Verification items for the finished model (mm, model axes). A direction names the side the tool comes from. Give positions to 0.01 mm unless a question says otherwise; leave off trailing zeros. Write each loop counter-clockwise with the first axis right and the second up, starting at its lowest first coordinate (ties: lowest second). Pieces come first, ordered by that corner, then holes. Notation, with made-up numbers: (79, 32) -> (138, 32) arc R31 ccw to (138, 65) -> close; hole circle Ø5 at (-39, -17.5). An arc over 180 degrees is marked (long way). Answer as CSV lines item,"result". Start each with the question number.
1) Material ranges on L1, parallel to Y at x = 34, z = -106.5; L2, parallel to Z at x = -22.5, y = 29, recorded low to high.
2) Sectioned sample at A-A on x = -19.5. Record the cut outline in (y, z), and give its area (3 significant figures).
3) Sectioned sample at B-B on y = 19. Record the cut outline in (x, z) (1 decimal).
4) Tool access check on faces 4 (the flat face through (0, 98, 48)), 5 (the flat face through (-31.8, -3.1, -146)), 6 (the flat face through (3.175, 98, 48)). Record the directions out of +Z, -Z, +X, -X, +Y, -Y that give a thin tool (end or side, any length) a straight path to the whole face; none if there is none.
5) Sectioned sample at C-C on z = 17. Record the cut outline in (x, y) (3 decimals), and give its area (3 significant figures).
6) Sectioned sample at D-D on z = -62.5. Record the cut outline in (x, y) (3 decimals), and give its area (3 significant figures).
7) Mould release check, pull along Y, two halves, no side actions. Record for faces 1 (the flat face through (31.7, -3.1, -146.1)), 2 (the flat face through (1.565, 80.451, 67.685)), 3 (the flat face through (-1, -6.35, 2)): released by +Y, released by -Y, zero draft, split by the parting line, or undercut.
8) Gauge pin test, flat ends, axial feed: pin 1 Ø2 at (x, y) = (-30.5, 119.5) entering from -Z; pin 2 Ø6 at (x, z) = (23, -87.5) entering from +Y; pin 3 Ø4 at (x, y) = (27.5, 221) entering from +Z. Record the tip position at first contact, or that the pin passes through.
```python
from build123d import *

# Parameters (mm, degrees)
F1_DEPTH = 6.35
F3_W     = 304.8
F3_H     = 6.35
F4_DEPTH = 76.2
F6_DEPTH = 3.175
F7_DEPTH = 3.175


with BuildPart() as f1:
    # F0 (on Front) → F1 (new body)
    with BuildSketch(Plane.XZ):
        Polygon((-25.4, -152.4), (25.4, -152.4), (38.1, -139.7), (38.1, 152.4), (-38.1, 152.4), (-38.1, -139.7), align=None)
    extrude(amount=F1_DEPTH)

    # F3 (on offset) → F4 (join)
    with BuildSketch(Plane.YZ.offset(38.1)):
        with Locations((152.4, 149.089498)):
            Rectangle(F3_W, F3_H)
    extrude(amount=-F4_DEPTH)

    # F5 (on Right) → F6 (join)
    with BuildSketch(Plane.YZ):
        Polygon((0, -66.648165), (212.562662, 145.914498), (158.681126, 145.914498), (0, -12.766628), align=None)
    extrude(amount=F6_DEPTH)

    # F5 (on Right) → F7 (join)
    with BuildSketch(Plane.YZ):
        Polygon((0, -66.648165), (212.562662, 145.914498), (158.681126, 145.914498), (0, -12.766628), align=None)
    extrude(amount=F7_DEPTH)


solid = f1.part
```
Ans:
1,L1,"y = -6.35 to 0"
1,L2,"z = 145.91 to 152.26"
2,outline,"(-6.35, -152.4) -> (0, -152.4) -> (0, 145.91) -> (304.8, 145.91) -> (304.8, 152.26) -> (0, 152.26) -> (0, 152.4) -> (-6.35, 152.4) -> close"
2,area,"3,870 mm²"
3,outline,"(-38.1, 145.9) -> (38.1, 145.9) -> (38.1, 152.3) -> (-38.1, 152.3) -> close; (0, -47.6) -> (3.2, -47.6) -> (3.2, 6.2) -> (0, 6.2) -> close"
4,face 4,"-Z, -X, +Y"
4,face 5,"-Z, -X, +Y, -Y"
4,face 6,"-Z, +X, +Y"
5,outline,"(-38.1, -6.35) -> (38.1, -6.35) -> (38.1, 0) -> (-38.1, 0) -> close; (0, 29.767) -> (3.175, 29.767) -> (3.175, 83.648) -> (0, 83.648) -> close"
5,area,"655 mm²"
6,outline,"(-38.1, -6.35) -> (38.1, -6.35) -> (38.1, 0) -> (3.175, 0) -> (3.175, 4.148) -> (0, 4.148) -> (0, 0) -> (-38.1, 0) -> close"
6,area,"497 mm²"
7,face 1,"zero draft"
7,face 2,"undercut"
7,face 3,"released by -Y"
8,pin 1,"stops at z = 145.91"
8,pin 2,"stops at y = 0"
8,pin 3,"stops at z = 152.26"
